Autodesk Inventor part; units mm, degrees
ref_plane "YZ Plane" through (0, 0, 0) normal (1, 0, 0) x (0, 1, 0)
ref_plane "XZ Plane" through (0, 0, 0) normal (0, 1, 0) x (-1, 0, 0)
ref_plane "XY Plane" through (0, 0, 0) normal (0, 0, 1) x (1, 0, 0)
sketch "Sketch1" plane through (0, 0, 0) normal (0, 0, 1) x (1, 0, 0)
  line L0 (-66.6872, 56.6432) -> (-66.6872, -62.4828)
  line L1 (-66.6872, -62.4828) -> (-4.7112, -62.4828)
  line L2 (-4.7112, -62.4828) -> (-4.7112, 56.6432)
  line L3 (-4.7112, 56.6432) -> (-66.6872, 56.6432)
  point P0 (0, 0)
  dimension "d0" = 119.126
  dimension "d1" = 61.976
extrude "Extrusion1" add sketch "Sketch1" along normal blind 6.604
sketch "Sketch2" plane through (0, 0, 6.604) normal (0, 0, 1) x (1, 0, 0)
  line L0 (-65.1652, 54.8612) -> (-6.2352, 54.8612)
  line L1 (-6.2352, 54.8612) -> (-6.2352, -60.9588)
  line L2 (-6.2352, -60.9588) -> (-65.1652, -60.9588)
  line L3 (-65.1652, -60.9588) -> (-65.1652, 54.8612)
  line L4 (-4.7112, -62.4828) -> (-4.7112, 56.6432)
  line L5 (-66.6872, -62.4828) -> (-4.7112, -62.4828)
  point P0 (0, 0)
  dimension "d4" = 115.82
  dimension "d5" = 58.93
  dimension "d6" = 1.524
  dimension "d7" = 1.524
extrude "Extrusion2" cut sketch "Sketch2" against normal blind 6.604
fillet "Fillet1" radius 1 4 edges at (-66.6872, -62.4828, 3.302) (-66.6872, 56.6432, 3.302) (-4.7112, 56.6432, 3.302) (-4.7112, -62.4828, 3.302)
properties part number "Smart Lock Box Middle Correct"
Check sheet for the modelled part. Datum: model origin and axes. Units: mm. A direction names the side the tool comes from. Round coordinates to 2 decimals unless told otherwise and drop trailing zeros. Order: outer loops, then holes, each group sorted by start corner. A loop starts at its lowest first (then second) coordinate and runs counter-clockwise, first axis right, second up. Notation, with made-up numbers: (54, 70.5) -> (107, 70.5) arc R11 ccw to (107, 85.5) -> close; hole circle Ø1 at (71.25, -17.75). An arc over 180 degrees is marked (long way). Use CSV: the item, a comma, the result in double quotes.
(1) Cross-section at A-A (x = -23.5). Record the boundary of the cut face in (y, z).
Worked out:
outline,"(-62.48, 0) -> (-60.96, 0) -> (-60.96, 6.6) -> (-62.48, 6.6) -> close; (54.86, 0) -> (56.64, 0) -> (56.64, 6.6) -> (54.86, 6.6) -> close"
(2) Material ranges on line 1 along X through (y, z) = (21, 5.5); line 2 along Y through (x, z) = (-34, 2), recorded low to high. Write a range as from..to.
Worked out:
line 1,"-66.69..-65.17, -6.24..-4.71"
line 2,"-62.48..-60.96, 54.86..56.64"
(3) Draft check along Y on faces 1 (the face through (-65.165, -4, 3)), 2 (the face through (-36, -62.483, 3)), 3 (the face through (-35, -60.959, 3)), 4 (the face through (-6, -3, 6.604)). Enter one of: pulls with the +Y half, pulls with the -Y half, needs draft (parallel to the pull), parting line crosses it, or undercut.
Worked out:
face 1,"undercut"
face 2,"pulls with the -Y half"
face 3,"undercut"
face 4,"needs draft"
(4) Tool access check on faces 5 (the face through (-4.711, -4, 3)), 6 (the face through (-36, 54.861, 3)). Record the directions out of +Z, -Z, +X, -X, +Y, -Y that give a thin tool (end or side, any length) a straight path to the whole face; none if there is none.
Worked out:
face 5,"+Z, -Z, +X, +Y, -Y"
face 6,"+Z, -Z"
(5) Cross-section at B-B (y = -48.5). Record the boundary of the cut face in (x, z), and give its area (3 significant figures).
Worked out:
outline,"(-66.69, 0) -> (-65.17, 0) -> (-65.17, 6.6) -> (-66.69, 6.6) -> close; (-6.24, 0) -> (-4.71, 0) -> (-4.71, 6.6) -> (-6.24, 6.6) -> close"
area,"20.1 mm²"
(6) Cross-section at C-C (z = 3.5). Record the boundary of the cut face in (x, y), and give its area (3 significant figures).
Worked out:
outline,"(-66.69, -61.48) arc R1 ccw to (-65.69, -62.48) -> (-5.71, -62.48) arc R1 ccw to (-4.71, -61.48) -> (-4.71, 55.64) arc R1 ccw to (-5.71, 56.64) -> (-65.69, 56.64) arc R1 ccw to (-66.69, 55.64) -> close; hole (-65.17, -60.96) -> (-6.24, -60.96) -> (-6.24, 54.86) -> (-65.17, 54.86) -> close"
area,"557 mm²"
